For this review, use the dimensioned drawing (mm, ordinates from the lowest corner) and the shaded views. Coordinates: 2 decimals unless noted, no trailing zeros. Order: outer loops, then holes, each group sorted by start corner. A loop starts at its lowest first (then second) coordinate and runs counter-clockwise, first axis right, second up. Notation, with made-up numbers: M 3,-34.5 L 47,-34.5 A19 cw 47,-2.5 Z; hole C 87.5,63 d11. An arc over 180 degrees is marked long. Use CSV: the item, a comma, the result in double quotes.
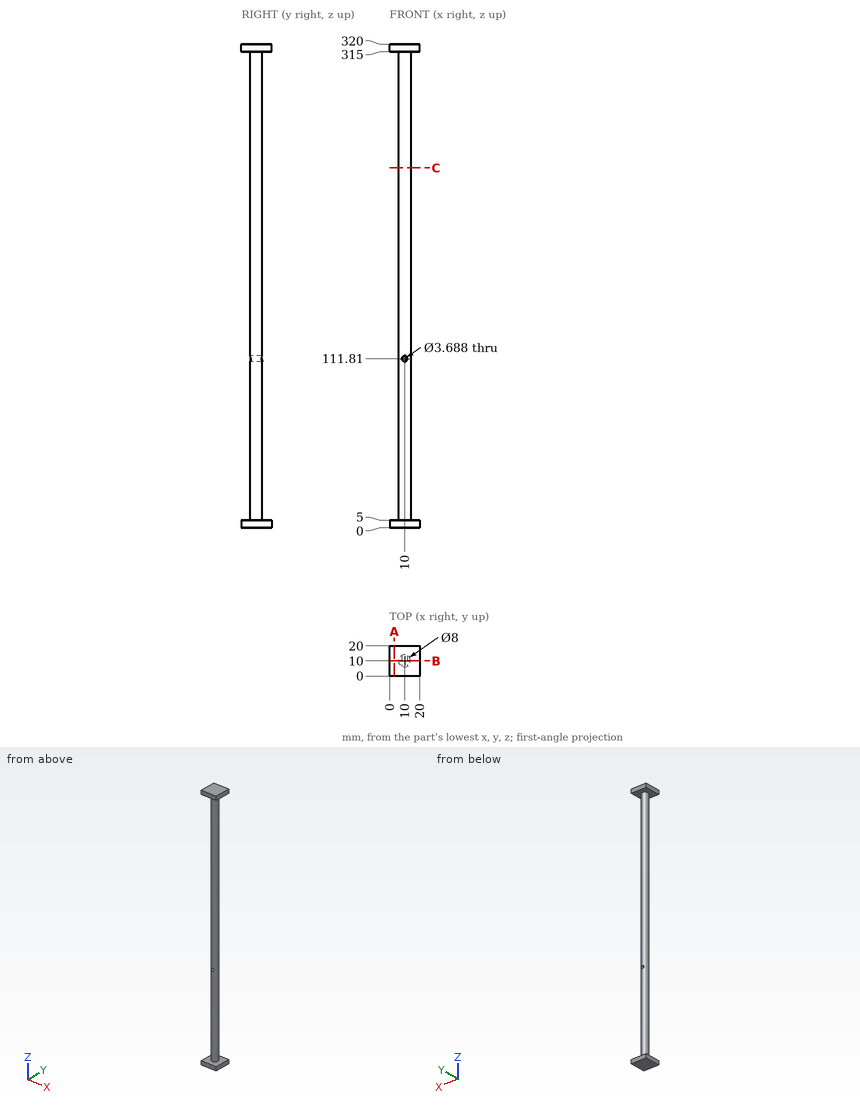
Item 1: To check wall thickness, follow line 1 along X through (y, z) = (10.25, 111.81); line 2 along Z through (x, y) = (10, 11.5); line 3 along Z through (x, y) = (18.5, 5.5). State the ranges of each line that lie inside material, in increasing order. Write a range as [from, to].
Solutions:
line 1,"[6.01, 8.16], [11.84, 13.99]"
line 2,"[0, 109.97], [113.65, 320]"
line 3,"[0, 5], [315, 320]"
Item 2: Add section C-C on z = 238. State the section outline as (x, y) points, and give its area (3 significant figures).
Solutions:
outline,"C 10,10 d8"
area,"50.3 mm^2"
Item 3: Clearance check with flat-ended pins moving along their axes: pin 1 Ø1 at (y, z) = (12.5, 111) entering from -X; pin 2 Ø10 at (y, z) = (8, 155) entering from -X; pin 3 Ø5 at (x, z) = (13.5, 41) entering from +Y; pin 4 Ø6 at (x, y) = (11.5, 7.5) entering from -Z. State where each tip first meets the part, or that it passes through.
Solutions:
pin 1,"x = 6.54"
pin 2,"x = 6"
pin 3,"y = 13.87"
pin 4,"z = 0"
Item 4: Add section A-A on x = 3.25. State the section outline as (y, z) points, and give its area (3 significant figures).
Solutions:
outline,"M 0,0 L 20,0 L 20,5 L 0,5 Z; M 0,315 L 20,315 L 20,320 L 0,320 Z"
area,"200 mm^2"
Item 5: Add section B-B on y = 10. State the section outline as (x, z) points, and give its area (3 significant figures).
Solutions:
outline,"M 0,0 L 20,0 L 20,5 L 14,5 L 14,315 L 20,315 L 20,320 L 0,320 L 0,315 L 6,315 L 6,5 L 0,5 Z; hole C 10,111.81 d3.69"
area,"2,670 mm^2"
